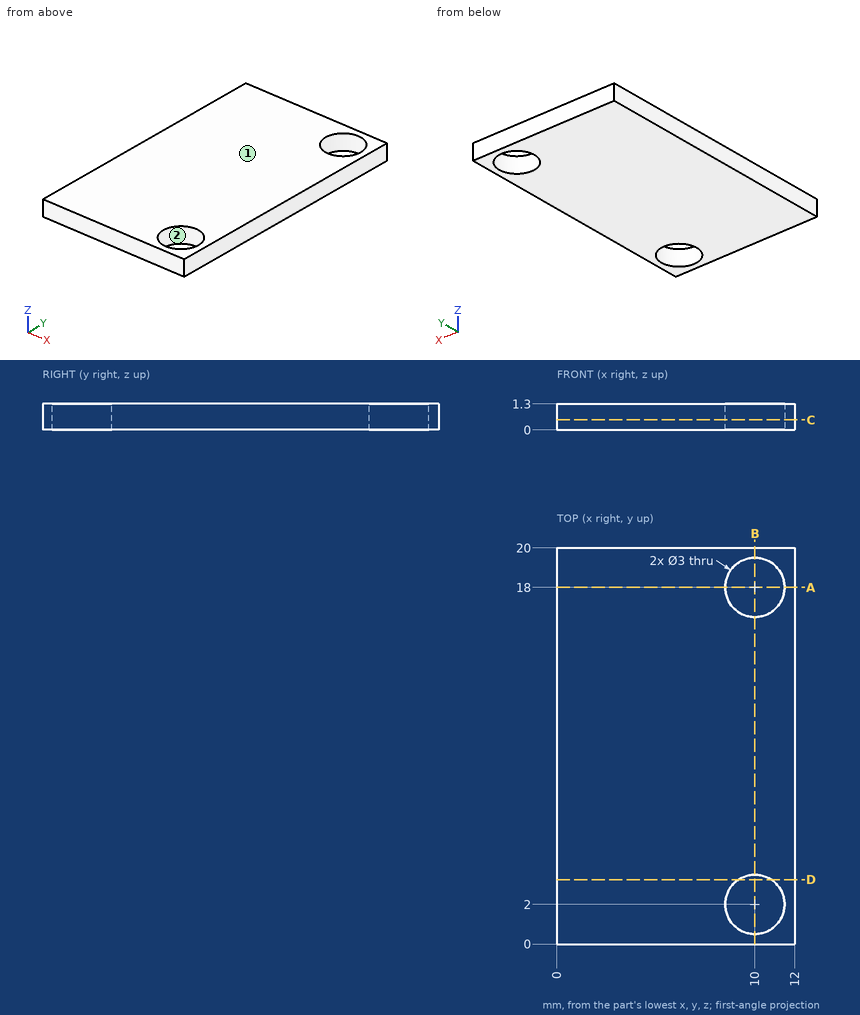
Print and shaded views of the part. All mm, measured from the part's lowest x, y and z. Give positions to 0.01 mm unless a question says otherwise; leave off trailing zeros. Write each loop counter-clockwise with the first axis right and the second up, starting at its lowest first coordinate (ties: lowest second). Pieces come first, ordered by that corner, then holes. Notation, with made-up numbers: (-2, 39) -> (45, 39) arc R33 ccw to (45, 74) -> close; hole circle Ø11 at (-38.5, -23.75). An arc over 180 degrees is marked (long way). Write item = value, one per line.
(1) Slice it at B-B, the plane x = 10. Give the cut face in (y, z).
Determined:
outline = (0, 0) -> (0.5, 0) -> (0.5, 1.3) -> (0, 1.3) -> close; (3.5, 0) -> (16.5, 0) -> (16.5, 1.3) -> (3.5, 1.3) -> close; (19.5, 0) -> (20, 0) -> (20, 1.3) -> (19.5, 1.3) -> close
(2) Slice it at C-C, the plane z = 0.5. Give the cut face in (x, y).
Determined:
outline = (0, 0) -> (12, 0) -> (12, 20) -> (0, 20) -> close; hole circle Ø3 at (10, 2); hole circle Ø3 at (10, 18)
(3) Slice it at D-D, the plane y = 3.25. Give the cut face in (x, z), then the cut area to 3 significant figures.
Determined:
outline = (0, 0) -> (9.17, 0) -> (9.17, 1.3) -> (0, 1.3) -> close; (10.83, 0) -> (12, 0) -> (12, 1.3) -> (10.83, 1.3) -> close
area = 13.4 mm2
(4) Probe line 1 along Y through (x, z) = (10, 1.05); line 2 along X through (y, z) = (18, 0.7); line 3 along Y through (x, z) = (9.5, 0.85). List the from-to ranges inside material, lowest first.
Determined:
line_1 = 0 to 0.5, 3.5 to 16.5, 19.5 to 20
line_2 = 0 to 8.5, 11.5 to 12
line_3 = 0 to 0.59, 3.41 to 16.59, 19.41 to 20
(5) Slice it at A-A, the plane y = 18. Give the cut face in (x, z), then the cut area to 3 significant figures.
Determined:
outline = (0, 0) -> (8.5, 0) -> (8.5, 1.3) -> (0, 1.3) -> close; (11.5, 0) -> (12, 0) -> (12, 1.3) -> (11.5, 1.3) -> close
area = 11.7 mm2
(6) Mould opens along X. For the marked faces 1 and 2 say: released by +X, released by -X, zero draft, split by the parting line, or undercut.
Determined:
face_1 = zero draft
face_2 = undercut
